The model under review builds one solid part; all positions refer to its coordinate system, in mm. A direction names the side the tool comes from. Give positions to 0.01 mm unless a question says otherwise; leave off trailing zeros. Loops run counter-clockwise (first coordinate to the right, second up) from the corner with the lowest first, then second, coordinate; pieces in that order, holes last. Notation, with made-up numbers: M 29.5,54 L 50.5,54 A15 cw 50.5,59 Z; hole C 8.25,65 d10. An arc over 180 degrees is marked long. Write item = value, one per line. Start each with the question number.
1. We need section A-A on x = 0. Give the boundary of the cut face in (y, z).
2. For faces 1 (the face through (0.066, 9.98, -10.028)), 2 (the face through (0, 0, -18)), 3 (the face through (3, 11.619, -12)), list the 3-axis set-ups (+Z, -Z, +X, -X, +Y, -Y) from which the entire face can be reached by the end or side of a thin tool; tool diameter is ignored.
3. We need section D-D on y = 13. Give the boundary of the cut face in (x, z).
4. For pin 1 (5 mm diameter, centred on y = 10, z = -11.5, fed in from +X); pin 2 (4 mm diameter, centred on y = 6, z = -13, fed in from +X); pin 3 (2.5 mm diameter, centred on x = 0, z = -11.53, fed in from +Y); pin 4 (3 mm diameter, centred on x = 3, z = -11, fed in from +Y), all flat-tipped, find the tip position at first contact; note any pin that passes through.
5. We need section C-C on z = -7.5. Give the boundary of the cut face in (x, y), then the cut area to 3 significant figures.
6. Draft analysis for pull direction Y (two halves, no side actions). For faces 4 (the face through (0.85, 13.71, -14.22)), 5 (the face through (0, 0, 0)), 6 (the face through (0.75, 8.21, -13.91)), state which applies: pulls with the +Y half, pulls with the -Y half, needs draft (parallel to the pull), parting line crosses it, or undercut.
7. We need section B-B on y = 8.25. Give the boundary of the cut face in (x, z).
8. Wall thickness on line 1 along Z through (x, y) = (0, 10.25); line 2 along X through (y, z) = (9.75, -11.5); line 3 along X through (y, z) = (13.5, -10.5): over which ranges is each line inside the solid? List them lowest first. Write a range as from..to.
from build123d import *

# Parameters (mm, degrees)
SKETCH1_R           = 5.5
BOSS_EXTRUDE1_DEPTH = 18


with BuildPart() as part:
    # Sketch1 → Boss-Extrude1 (new body)
    with BuildSketch(Plane.XY):
        Circle(SKETCH1_R)
    extrude(amount=-BOSS_EXTRUDE1_DEPTH)

    # Sketch3 → Revolve1 (revolve)
    with BuildSketch(Plane(origin=(0, 0, 0), x_dir=(0, 0, -1), z_dir=(1, 0, 0))):
        Polygon((13.026280971, 14.539629518), (14.13388163, 14.539629518), (14.897758762, 11.619086594), (14.026280971, 11.619086594), (14.026280971, 0.039629518), (13.026280971, 0.039629518), align=None)
    revolve(axis=Axis((0, 14.539629518, -11.526280971), (0, -1, 0)))


solid = part.part
Final values:
q1.outline = M -5.5,-18 L 5.5,-18 L 5.5,-14.03 L 11.62,-14.03 L 11.62,-14.9 L 14.54,-14.13 L 14.54,-13.03 L 5.5,-13.03 L 5.5,-10.03 L 14.54,-10.03 L 14.54,-8.92 L 11.62,-8.15 L 11.62,-9.03 L 5.5,-9.03 L 5.5,0 L -5.5,0 Z
q2.face_1 = +Y
q2.face_2 = -Z, +X, -X, +Y, -Y
q2.face_3 = none
q3.outline = C 0,-11.53 d6.02; hole C 0,-11.53 d3
q4.pin_1 = 3.37
q4.pin_2 = 3.77
q4.pin_3 = 5.5
q4.pin_4 = 14.54
q5.outline = C 0,0 d11
q5.area = 95.0 mm²
q6.face_4 = pulls with the +Y half
q6.face_5 = needs draft
q6.face_6 = undercut
q7.outline = C 0,-11.53 d5; hole C 0,-11.53 d3
q8.line_1 = -14.03..-13.03, -10.03..-9.03
q8.line_2 = -2.5..-1.5, 1.5..2.5
q8.line_3 = -2.69..-1.09, 1.09..2.69
